Part model, mm, in its own coordinate system. A direction names the side the tool comes from. Give positions to 0.01 mm unless a question says otherwise; leave off trailing zeros. Write each loop counter-clockwise with the first axis right and the second up, starting at its lowest first coordinate (ties: lowest second). Pieces come first, ordered by that corner, then holes. Notation, with made-up numbers: M 86,9 L 100,9 A14 ccw 100,27 Z; hole C -12.75,77 d11. An arc over 180 degrees is marked long. Answer as CSV lines item,"result". Start each with the question number.
Item 1: Pin check, flat tips, straight feed: pin 1 (1.8 mm diameter, centred on y = 125.5, z = 1, fed in from +X); pin 2 (2.5 mm diameter, centred on y = 124.16, z = 0, fed in from -X); pin 3 (10 mm diameter, centred on x = 130, y = 13, fed in from +Z); pin 4 (7 mm diameter, centred on y = 18, z = 92, fed in from -X). Stop position of each tip, or through.
Item 2: Band-saw the part on A-A, the plane x = 43.5. List the corners of the cut face in (y, z), then the cut area to 3 significant figures.
Item 3: Two-plate mould, pull along X, no slides. Class faces 1 (the flat face through (152.298, 14, 81)), 2 (the flat face through (5, -121, 0)), 3 (the flat face through (155, -11.5, 63)): +X half, -X half, draft (parallel to the pull), parting line (faces both ways), or undercut.
Item 4: Band-saw the part on B-B, the plane y = 0. List the corners of the cut face in (x, z).
Item 5: Band-saw the part on C-C, the plane z = 85.5. List the corners of the cut face in (x, y), then the cut area to 3 significant figures.
Item 6: Band-saw the part on D-D, the plane x = 101. List the corners of the cut face in (y, z), then the cut area to 3 significant figures.
Item 7: 3-axis set-ups, long thin cutter, end or side, ignore diameter. For faces 4 (the flat face through (152.298, -13, 81)), 5 (the flat face through (155.298, 0, 81)), 6 (the flat face through (154, 15, 62)), 7 (the flat face through (155, 11.5, 63)): which of +Z, -Z, +X, -X, +Y, -Y reach the whole face in a straight line?
Item 8: Wall check: L1, parallel to Y at x = 1.15, z = 0; L2, parallel to Y at x = 3.2, z = 0; L3, parallel to Y at x = 155, z = 135. Give the ranges that are in metal, low to high. Write a range as from..to.
from build123d import *

# Parameters (mm, degrees)
SKETCH_1_R                = 115
SKETCH_1_R_2              = 105
EXTRUDE_1_DEPTH           = 5
SKETCH_4_R                = 2.5
CUT_EXTRUDE_1_DEPTH       = 33.934862746
EXTRUDE_2_DEPTH           = 5
HOLE_WIZARD_1_D           = 4.5
HOLE_WIZARD_1_CBORE_D     = 6
HOLE_WIZARD_1_CBORE_DEPTH = 3
SKETCH_9_R                = 2.25
SKETCH_9_R_2              = 1.9
EXTRUDE_3_DEPTH           = 5
EXTRUDE_4_DEPTH           = 5
HOLE_WIZARD_2_D           = 4.5
HOLE_WIZARD_2_CBORE_D     = 6
HOLE_WIZARD_2_CBORE_DEPTH = 3
SKETCH_13_R               = 2.25
SKETCH_13_R_2             = 1.9
EXTRUDE_5_DEPTH           = 5
SKETCH_14_W               = 562.038590931
SKETCH_14_H               = 462.09177453
CUT_EXTRUDE_4_DEPTH       = 163.29776757
SKETCH_15_W               = 637.223239982
SKETCH_15_H               = 375.31186697
CUT_EXTRUDE_5_DEPTH       = 202.710100717


with BuildPart() as part:
    # 草图1 → 凸台-拉伸1 (new body, symmetric)
    with BuildSketch(Plane.XY):
        Circle(SKETCH_1_R)
        Circle(SKETCH_1_R_2, mode=Mode.SUBTRACT)
    extrude(amount=EXTRUDE_1_DEPTH, both=True)

    # 扫描1: sweep along a path in 草图2
    with BuildLine(Plane(origin=(0, 0, 0), x_dir=(1, 0, 0), z_dir=(0, 1, 0))) as sweep_1_path:
        Line((-130, -355), (-156.694693778, -281.656931626))
        ThreePointArc((-156.694693778, -281.656931626), (-157.1458451, -279.97321197), (-157.29776757, -278.236730193))
        Line((-157.29776757, -278.236730193), (-157.29776757, -10))
        ThreePointArc((-157.29776757, -10), (-154.368835382, -2.928932188), (-147.29776757, 0))
        Line((-147.29776757, 0), (-115, 0))
        Line((-115, 0), (-106.681302201, 0))
    # 草图3 → 扫描1 (sweep)
    with BuildSketch(Plane(origin=(-130, 0, 355), x_dir=(0.939692621, 0, -0.342020143), z_dir=(0.342020143, 0, 0.939692621))):
        Polygon((-5, -15), (5, -15), (5, -11.5), (2, -11.5), (2, 11.5), (5, 11.5), (5, 15), (-5, 15), align=None)
    sweep_1 = sweep(path=sweep_1_path.line)

    # 草图4 → 切除-拉伸1 (cut, through all)
    with BuildSketch(Plane(origin=(-227.008304281, 0, 82.624265689), x_dir=(-0.342020143, 0, -0.939692621), z_dir=(0.939692621, 0, -0.342020143))):
        with Locations((-274.128261747, 6.75)):
            Circle(SKETCH_4_R)
        with Locations((-274.128261747, -6.75)):
            Circle(SKETCH_4_R)
    cut_extrude_1 = extrude(amount=-CUT_EXTRUDE_1_DEPTH, mode=Mode.SUBTRACT)

    # 镜向1: 扫描1, 切除-拉伸1 across plane
    add(sweep_1.mirror(Plane(origin=(0, 0, 0), x_dir=(0, 0, 1), z_dir=(1, 0, 0))))
    add(cut_extrude_1.mirror(Plane(origin=(0, 0, 0), x_dir=(0, 0, 1), z_dir=(1, 0, 0))), mode=Mode.SUBTRACT)

    # 草图6 → 凸台-拉伸2 (add, symmetric)
    with BuildSketch(Plane(origin=(0, 0, 0), x_dir=(0, 0, -1), z_dir=(1, 0, 0))):
        with BuildLine():
            Line((-5, 115), (-5, 125))
            ThreePointArc((-5, 125), (0, 130), (5, 125))
            Line((5, 125), (5, 115))
            Line((5, 115), (5, 112.136445143))
            Line((5, 112.136445143), (-5, 112.136445143))
            Line((-5, 112.136445143), (-5, 115))
        make_face()
    extrude_2 = extrude(amount=EXTRUDE_2_DEPTH, both=True)

    # 镜向2: 凸台-拉伸2 across plane
    add(extrude_2.mirror(Plane.ZX))

    # 孔1 (through all)
    with Locations(Plane(origin=(5, 0, 0), x_dir=(0, 0, -1), z_dir=(1, 0, 0))):
        with Locations((0, 124.156343107), (0, -125)):
            CounterBoreHole(HOLE_WIZARD_1_D / 2, HOLE_WIZARD_1_CBORE_D / 2, HOLE_WIZARD_1_CBORE_DEPTH)

    # 草图9 → 凸台-拉伸3 (add)
    with BuildSketch(Plane.ZY.offset(5)):
        with Locations((0, 124.156343107)):
            Circle(SKETCH_9_R)
        with Locations((0, 124.156343107)):
            Circle(SKETCH_9_R_2, mode=Mode.SUBTRACT)
        with Locations((0, -125)):
            Circle(SKETCH_9_R)
        with Locations((0, -125)):
            Circle(SKETCH_9_R_2, mode=Mode.SUBTRACT)
    extrude(amount=-EXTRUDE_3_DEPTH)

    # 草图10 → 凸台-拉伸4 (add, symmetric)
    with BuildSketch(Plane.XY.offset(155)):
        with BuildLine():
            Line((-162.29776757, 15), (-152.29776757, 15))
            Line((-152.29776757, 15), (-152.29776757, 20))
            ThreePointArc((-152.29776757, 20), (-157.29776757, 25), (-162.29776757, 20))
            Line((-162.29776757, 20), (-162.29776757, 15))
        make_face()
        with BuildLine():
            Line((-152.29776757, -15), (-152.29776757, -20))
            ThreePointArc((-152.29776757, -20), (-157.29776757, -25), (-162.29776757, -20))
            Line((-162.29776757, -20), (-162.29776757, -15))
            Line((-162.29776757, -15), (-152.29776757, -15))
        make_face()
        with BuildLine():
            Line((162.29776757, -15), (152.29776757, -15))
            Line((152.29776757, -15), (152.29776757, -20))
            ThreePointArc((152.29776757, -20), (157.29776757, -25), (162.29776757, -20))
            Line((162.29776757, -20), (162.29776757, -15))
        make_face()
        with BuildLine():
            Line((152.29776757, 15), (152.29776757, 20))
            ThreePointArc((152.29776757, 20), (157.29776757, 25), (162.29776757, 20))
            Line((162.29776757, 20), (162.29776757, 15))
            Line((162.29776757, 15), (152.29776757, 15))
        make_face()
    extrude(amount=EXTRUDE_4_DEPTH, both=True)

    # 孔2 (through all)
    with Locations(Plane.XY.offset(160)):
        with Locations((-157.29776757, 20), (-157.29776757, -20), (157.29776757, 20), (157.29776757, -20)):
            CounterBoreHole(HOLE_WIZARD_2_D / 2, HOLE_WIZARD_2_CBORE_D / 2, HOLE_WIZARD_2_CBORE_DEPTH)

    # 草图13 → 凸台-拉伸5 (add)
    with BuildSketch(Plane(origin=(0, 0, 150), x_dir=(-1, 0, 0), z_dir=(0, 0, -1))):
        with Locations((-157.29776757, 20)):
            Circle(SKETCH_13_R)
        with Locations((-157.29776757, 20)):
            Circle(SKETCH_13_R_2, mode=Mode.SUBTRACT)
        with Locations((-157.29776757, -20)):
            Circle(SKETCH_13_R)
        with Locations((-157.29776757, -20)):
            Circle(SKETCH_13_R_2, mode=Mode.SUBTRACT)
        with Locations((157.29776757, -20)):
            Circle(SKETCH_13_R)
        with Locations((157.29776757, -20)):
            Circle(SKETCH_13_R_2, mode=Mode.SUBTRACT)
        with Locations((157.29776757, 20)):
            Circle(SKETCH_13_R)
        with Locations((157.29776757, 20)):
            Circle(SKETCH_13_R_2, mode=Mode.SUBTRACT)
    extrude(amount=-EXTRUDE_5_DEPTH)

    # 草图14 → 切除-拉伸4 (cut, through all)
    with BuildSketch(Plane(origin=(0, 0, 0), x_dir=(0, 0, -1), z_dir=(1, 0, 0))):
        with Locations((-153.139864812, -31.152254463)):
            Rectangle(SKETCH_14_W, SKETCH_14_H)
    extrude(amount=-CUT_EXTRUDE_4_DEPTH, mode=Mode.SUBTRACT)

    # 草图15 → 切除-拉伸5 (cut, through all)
    with BuildSketch(Plane.XY.offset(155)):
        Rectangle(SKETCH_15_W, SKETCH_15_H)
    extrude(amount=CUT_EXTRUDE_5_DEPTH, mode=Mode.SUBTRACT)


solid = part.part
Output:
1,pin 1,"x = 2"
1,pin 2,"through"
1,pin 3,"z = 5"
1,pin 4,"x = 152.3"
2,outline,"M -106.46,-5 L -95.57,-5 L -95.57,5 L -106.46,5 Z; M 95.57,-5 L 106.46,-5 L 106.46,5 L 95.57,5 Z"
2,area,"218 mm²"
3,face 1,"-X half"
3,face 2,"+X half"
3,face 3,"undercut"
4,outline,"M 105,-5 L 147.3,-5 A15 ccw 162.3,10 L 162.3,155 L 155.3,155 L 155.3,10 A8 cw 147.3,2 L 115,2 L 115,5 L 105,5 Z"
5,outline,"M 152.3,-15 L 162.3,-15 L 162.3,15 L 152.3,15 L 152.3,11.5 L 155.3,11.5 L 155.3,-11.5 L 152.3,-11.5 Z"
5,area,"231 mm²"
6,outline,"M -54.99,-5 L -28.71,-5 L -28.71,5 L -54.99,5 Z; M 28.71,-5 L 54.99,-5 L 54.99,5 L 28.71,5 Z"
6,area,"526 mm²"
7,face 4,"+Z, -X, +Y, -Y"
7,face 5,"+Z, -X"
7,face 6,"-Z, +X, +Y"
7,face 7,"+Z"
8,L1,"-130..-127.25, -122.75..-104.99, 104.99..121.91, 126.41..130"
8,L2,"-130..-128, -122..-104.95, 104.95..121.16, 127.16..130"
8,L3,"-15..-11.5, 11.5..15"
